CAD build for the part. Positions are in the model's coordinates, mm. A direction names the side the tool comes from. Coordinates: 2 decimals unless noted, no trailing zeros. Order: outer loops, then holes, each group sorted by start corner. A loop starts at its lowest first (then second) coordinate and runs counter-clockwise, first axis right, second up. Notation, with made-up numbers: (58, 53) - (108, 53) arc R28 cw to (108, 91) - close; hole circle Ø8 at (81.25, 34.5). An arc over 180 degrees is marked (long way). Return JSON: item names as keys, results as strings.
from build123d import *

# Parameters (mm, degrees)
F1_DEPTH = 4
F2_R     = 1.5
F3_R     = 1.6
F4_DEPTH = 4.001
F5_R     = 34.9
F6_DEPTH = 4.001


# Not quite as in the source:
# - a feature names something its author has since deleted; it is built from what else it names


with BuildPart() as f1:
    # F0 (on Top) → F1 (new body)
    with BuildSketch(Plane.XY):
        with BuildLine():
            ThreePointArc((-39.0789468534, 31.1903176135), (-41.1995846792, 28.3300939331), (-43.1112914302, 25.3262028584))
            ThreePointArc((-43.1112914302, 25.3262028584), (3.3909583102, -49.8848814947), (39.2874210825, 30.9273106604))
            ThreePointArc((39.2874210825, 30.9273106604), (23.4196994292, 44.1759853161), (3.5489706102, 49.8738890363))
            Line((3.5489706102, 49.8738890363), (3.5489706102, 39.2354845469))
            ThreePointArc((3.5489706102, 39.2354845469), (0, 35.6), (-3.5489706102, 39.2354845469))
            Line((-3.5489706102, 39.2354845469), (-3.5489706102, 49.8738890363))
            ThreePointArc((-3.5489706102, 49.8738890363), (-19.9954983208, 45.8277213802), (-34.1476646001, 36.5231023102))
            ThreePointArc((-34.1476646001, 36.5231023102), (-36.7102683781, 33.9463723482), (-39.0789468534, 31.1903176135))
        make_face()
        with BuildLine():
            Line((-36.0538297274, -7.1563580217), (-16.4297758662, 26.0448529843))
            ThreePointArc((-16.4297758662, 26.0448529843), (-12.9279784785, 29.4992312077), (-8.176710299, 30.7723237188))
            Line((-8.176710299, 30.7723237188), (8.4702026349, 30.8290335362))
            ThreePointArc((8.4702026349, 30.8290335362), (13.1364940427, 29.5958615472), (16.5612188168, 26.1949427186))
            Line((16.5612188168, 26.1949427186), (35.9620596652, -7.1371930753))
            ThreePointArc((35.9620596652, -7.1371930753), (37.2684771199, -12.0112511492), (35.9293854445, -16.8764337932))
            Line((35.9293854445, -16.8764337932), (27.4589141067, -31.2073110011))
            ThreePointArc((27.4589141067, -31.2073110011), (23.957116719, -34.6616892246), (19.2058485395, -35.9347817357))
            Line((19.2058485395, -35.9347817357), (-19.3610626759, -36.0661648035))
            ThreePointArc((-19.3610626759, -36.0661648035), (-24.1774760593, -34.793319721), (-27.7123796465, -31.2829879542))
            Line((-27.7123796465, -31.2829879542), (-36.0865039481, -16.8955987396))
            ThreePointArc((-36.0865039481, -16.8955987396), (-37.3929214028, -12.0215406656), (-36.0538297274, -7.1563580217))
        make_face(mode=Mode.SUBTRACT)
    extrude(amount=F1_DEPTH)

    # F2
    f2_edges = [f1.edges().sort_by_distance(p)[0] for p in [
        (39.287421, 30.927311, 2),
        (3.548971, 49.873889, 2),
    ]]
    fillet(f2_edges, radius=F2_R)

    # F3 (on face) → F4 (cut, through all)
    with BuildSketch(Plane.XY.offset(4)):
        with Locations((0, 45.69)):
            Circle(F3_R)
        with Locations((-45.69, 0)):
            Circle(F3_R)
        with Locations((0, -45.69)):
            Circle(F3_R)
        with Locations((45.69, 0)):
            Circle(F3_R)
    extrude(amount=-F4_DEPTH, mode=Mode.SUBTRACT)

    # F5 (on face) → F6 (cut, through all)
    with BuildSketch(Plane.XY.offset(4)):
        with Locations((0, -5.7566108276)):
            Circle(F5_R)
    extrude(amount=-F6_DEPTH, mode=Mode.SUBTRACT)


solid = f1.part
Item 1: Band-saw the part on C-C, the plane z = 1.9. Count the separate pieces of the cut face and the enclosed holes in it, then the cut area to 3 significant figures.
Findings below:
{"separate pieces": "1", "enclosed holes": "4", "area": "3,660 mm²"}
Item 2: Which spindle directions (+Z, -Z, +X, -X, +Y, -Y) get a long thin tool onto all of the face, cutting with end or side? Do faces 1 (the flat face through (3.549, 44, 2)), 2 (the flat face through (-31.84, -24.19, 1.97)), 3 (the flat face through (22, 23, 4)). Say none if no direction does.
Findings below:
{"face 1": "+Z, -Z, +Y", "face 2": "+Z, -Z", "face 3": "+Z, +X, -X, +Y, -Y"}
Item 3: Band-saw the part on B-B, the plane x = 25.5. List the corners of the cut face in (y, z), then the cut area to 3 significant figures.
Findings below:
{"outline": "(-43.01, 0) - (-33.56, 0) - (-33.56, 4) - (-43.01, 4) - close; (18.07, 0) - (43.01, 0) - (43.01, 4) - (18.07, 4) - close", "area": "138 mm²"}
Item 4: Drop flat-ended pins along their axis: P1, Ø1.2, axis at y = 44, z = 2.5, coming from the +X side; P2, Ø1, axis at y = -35.5, z = 2.5, coming from the +X side. Give the stop position or say it passes through.
Findings below:
{"P1": "stops at x = 24.83", "P2": "stops at x = 35.71"}
Item 5: Wall check: L1, parallel to Y at x = 0, z = 1.7; L2, parallel to X at y = 28.5, z = 0.5; L3, parallel to X at y = -15, z = 1.65. Give the ranges that are in metal, low to high. Write a range as [from, to].
Findings below:
{"L1": "y = [-50, -47.29], [-44.09, -40.66], [30.8, 35.6]", "L2": "x = [-41.08, -14.36], [14.67, 41.08]", "L3": "x = [-47.7, -36.93], [36.78, 47.7]"}
Item 6: Mould opens along Y. For faces 4 (the cylindrical face through (24.017, -34.627, 1.972)), 5 (the flat face through (22, 23, 0)) say: released by +Y, released by -Y, zero draft, split by the parting line, or undercut.
Findings below:
{"face 4": "undercut", "face 5": "zero draft"}
Item 7: Band-saw the part on A-A, the plane y = -14.5. List the corners of the cut face in (x, z), then the cut area to 3 significant figures.
Findings below:
{"outline": "(-47.85, 0) - (-37.08, 0) - (-37.08, 4) - (-47.85, 4) - close; (36.93, 0) - (47.85, 0) - (47.85, 4) - (36.93, 4) - close", "area": "86.8 mm²"}
Item 8: Band-saw the part on D-D, the plane y = 0. List the corners of the cut face in (x, z), then the cut area to 3 significant figures.
Findings below:
{"outline": "(-50, 0) - (-47.29, 0) - (-47.29, 4) - (-50, 4) - close; (-44.09, 0) - (-34.42, 0) - (-34.42, 4) - (-44.09, 4) - close; (34.42, 0) - (44.09, 0) - (44.09, 4) - (34.42, 4) - close; (47.29, 0) - (50, 0) - (50, 4) - (47.29, 4) - close", "area": "99.0 mm²"}
